Check sheet for the modelled part. Datum: model origin and axes. Units: mm. A direction names the side the tool comes from. Give positions to 0.01 mm unless a question says otherwise; leave off trailing zeros. Order: outer loops, then holes, each group sorted by start corner. A loop starts at its lowest first (then second) coordinate and runs counter-clockwise, first axis right, second up. Notation, with made-up numbers: (30.5, 88) -> (78.5, 88) arc R33 cw to (78.5, 118) -> close; hole circle Ø5 at (47, -36). An arc over 180 degrees is marked (long way). Write each question's results on one line, items separated by ' | '.
Autodesk Inventor part; units mm, degrees
ref_plane "YZ Plane" through (0, 0, 0) normal (1, 0, 0) x (0, 1, 0)
ref_plane "XZ Plane" through (0, 0, 0) normal (0, 1, 0) x (-1, 0, 0)
ref_plane "XY Plane" through (0, 0, 0) normal (0, 0, 1) x (1, 0, 0)
sketch "Boceto1" plane through (0, 0, 0) normal (0, 1, 0) x (-1, 0, 0)
  line L0 (17.5, 45) -> (-17.5, 45)
  line L1 (-22.5, 40) -> (-22.5, -40)
  line L2 (-17.5, -45) -> (17.5, -45)
  line L3 (22.5, -40) -> (22.5, 40)
  line L4 (22.5, 45) -> (-22.5, -45) construction
  line L5 (-22.5, 45) -> (22.5, -45) construction
  arc A0 (22.5, 40) -> (17.5, 45) centre (17.5, 40) ccw
  arc A1 (-17.5, 45) -> (-22.5, 40) centre (-17.5, 40) ccw
  arc A2 (-22.5, -40) -> (-17.5, -45) centre (-17.5, -40) ccw
  arc A3 (17.5, -45) -> (22.5, -40) centre (17.5, -40) ccw
  point P0 (0, 0)
  dimension "d0" = 45
  dimension "d1" = 90
  dimension "d2" = 5
extrude "Extrusión1" add sketch "Boceto1" along normal blind 10
sketch "Boceto2" plane through (0, 10, 0) normal (0, 1, 0) x (1, 0, 0)
  arc A0 (17.5, -45) -> (22.5, -40) centre (17.5, -40) ccw
  line L0 (22.5, -40) -> (22.5, 40)
  arc A1 (22.5, 40) -> (17.5, 45) centre (17.5, 40) ccw
  line L1 (17.5, 45) -> (-17.5, 45)
  arc A2 (-17.5, 45) -> (-22.5, 40) centre (-17.5, 40) ccw
  line L2 (-22.5, 40) -> (-22.5, -40)
  arc A3 (-22.5, -40) -> (-17.5, -45) centre (-17.5, -40) ccw
  line L3 (-17.5, -45) -> (17.5, -45)
  arc A4 (-21.5, -40) -> (-17.5, -44) centre (-17.5, -40) ccw
  line L4 (-21.5, -40) -> (-21.5, 40)
  arc A5 (-17.5, 44) -> (-21.5, 40) centre (-17.5, 40) ccw
  line L5 (-17.5, 44) -> (17.5, 44)
  arc A6 (21.5, 40) -> (17.5, 44) centre (17.5, 40) ccw
  line L6 (21.5, 40) -> (21.5, -40)
  arc A7 (17.5, -44) -> (21.5, -40) centre (17.5, -40) ccw
  line L7 (17.5, -44) -> (-17.5, -44)
  line L8 (-20.5, 40) -> (-20.5, -40)
  arc A8 (-20.5, -40) -> (-17.5, -43) centre (-17.5, -40) ccw
  line L9 (-17.5, -43) -> (17.5, -43)
  arc A9 (17.5, -43) -> (20.5, -40) centre (17.5, -40) ccw
  line L10 (20.5, -40) -> (20.5, 40)
  arc A10 (20.5, 40) -> (17.5, 43) centre (17.5, 40) ccw
  line L11 (17.5, 43) -> (-17.5, 43)
  arc A11 (-17.5, 43) -> (-20.5, 40) centre (-17.5, 40) ccw
  point P0 (0, 0)
  dimension "d5" = 1
  dimension "d6" = 1
extrude "Extrusión2" cut sketch "Boceto2" against normal blind 2 contours L4 A5 L5 A6 L6 A7 L7 A4
sketch "Boceto3" plane through (0, 10, 0) normal (0, 1, 0) x (1, 0, 0)
  line L0 (17.5, 43) -> (-17.5, 43)
  arc A0 (-17.5, 43) -> (-20.5, 40) centre (-17.5, 40) ccw
  line L1 (-20.5, 40) -> (-20.5, -40)
  arc A1 (-20.5, -40) -> (-17.5, -43) centre (-17.5, -40) ccw
  line L2 (-17.5, -43) -> (17.5, -43)
  arc A2 (17.5, -43) -> (20.5, -40) centre (17.5, -40) ccw
  line L3 (20.5, -40) -> (20.5, 40)
  arc A3 (20.5, 40) -> (17.5, 43) centre (17.5, 40) ccw
  point P0 (0, 0)
extrude "Extrusión3" cut sketch "Boceto3" against normal blind 7
sketch "Boceto4" plane through (0, 3, 0) normal (0, 1, 0) x (1, 0, 0)
  circle A0 centre (0, 0) radius 2
  circle A1 centre (0, 0) radius 1.1
  dimension "d11" = 4
  dimension "d12" = 2.2
extrude "Extrusión4" add sketch "Boceto4" along normal blind 5.4
fillet "Empalme1" radius 2 1 edges at (-2, 3, 0)
sketch "Boceto5" plane through (0, 3, 0) normal (0, 1, 0) x (1, 0, 0)
  line L0 (17.5, -43) -> (-17.5, -43) construction
  line L1 (0, -43) -> (0, -37.1) construction
  line L2 (-17.5, 43) -> (17.5, 43) construction
  line L3 (0, 43) -> (0, 37.1) construction
  circle A0 centre (0, -37.1) radius 2
  circle A1 centre (0, -37.1) radius 1.1
  circle A2 centre (0, 37.1) radius 2
  circle A3 centre (0, 37.1) radius 1.1
  point P0 (0, 0)
  dimension "d16" = 5.9
  dimension "d17" = 5.9
  dimension "d18" = 4
  dimension "d19" = 2.2
  dimension "d20" = 4
  dimension "d21" = 2.2
extrude "Extrusión5" add sketch "Boceto5" along normal blind 5.4
fillet "Empalme2" radius 2 2 edges at (-2, 3, 37.1) (-2, 3, -37.1)
sketch "Sketch10" plane through (17.5, 0, -45) normal (0, 0, -1) x (-1, 0, 0)
  line L0 (-3.0024, 10) -> (14.9976, 10)
  line L1 (14.9976, 10) -> (14.9976, 7)
  line L2 (14.9976, 7) -> (-3.0024, 7)
  line L3 (-3.0024, 7) -> (-3.0024, 10)
  point P0 (17.5, 0)
  dimension "d37" = 18
  dimension "d38" = 3
extrude "Extrusion10" cut sketch "Sketch10" against normal blind 5
properties part number "Pieza_baja"
1. Material ranges on probe 1 along X at (y, z) = (5, 0); probe 2 along Z at (x, y) = (10, 3.75); probe 3 along X at (y, z) = (9.5, -0.5), recorded low to high. Write a range as from..to.
Verdict:
probe 1: x = -22.5..-20.5, -2..-1.1, 1.1..2, 20.5..22.5 | probe 2: z = -45..-43, 43..45 | probe 3: x = -22.5..-21.5, 21.5..22.5
2. Gauge pin test, flat ends, axial feed: pin 1 Ø2.5 at (x, z) = (0, -37.5) entering from +Y; pin 2 Ø20.5 at (x, z) = (-9.5, -18) entering from +Y; pin 3 Ø2.5 at (x, z) = (16, -42.5) entering from +Y. Record the tip position at first contact, or that the pin passes through.
Verdict:
pin 1: stops at y = 8.4 | pin 2: stops at y = 3 | pin 3: stops at y = 7
3. Mould release check, pull along X, two halves, no side actions. Record for faces 4 (the flat face through (-22.5, 5, -1)), 5 (the flat face through (22.5, 5, 1)), 6 (the cylindrical face through (0.923, 6.676, 35.326)): +X half, -X half, draft (parallel to the pull), parting line (faces both ways), or undercut.
Verdict:
face 4: -X half | face 5: +X half | face 6: undercut
4. Section check A-A on y = 6. Record the cut outline in (x, z).
Verdict:
outline: (-22.5, -40) arc R5 ccw to (-17.5, -45) -> (17.5, -45) arc R5 ccw to (22.5, -40) -> (22.5, 40) arc R5 ccw to (17.5, 45) -> (-17.5, 45) arc R5 ccw to (-22.5, 40) -> close; circle Ø4 at (0, -37.1); circle Ø4 at (0, 0); circle Ø4 at (0, 37.1); hole (-20.5, -40) arc R3 ccw to (-17.5, -43) -> (17.5, -43) arc R3 ccw to (20.5, -40) -> (20.5, 40) arc R3 ccw to (17.5, 43) -> (-17.5, 43) arc R3 ccw to (-20.5, 40) -> close; hole circle Ø2.2 at (0, -37.1); hole circle Ø2.2 at (0, 0); hole circle Ø2.2 at (0, 37.1)
5. Section check C-C on x = -15.5. Record the cut outline in (y, z).
Verdict:
outline: (0, -45) -> (10, -45) -> (10, -44) -> (8, -44) -> (8, -43) -> (3, -43) -> (3, 43) -> (8, 43) -> (8, 44) -> (10, 44) -> (10, 45) -> (0, 45) -> close
6. Section check D-D on z = 25. Record the cut outline in (x, y).
Verdict:
outline: (-22.5, 0) -> (22.5, 0) -> (22.5, 10) -> (21.5, 10) -> (21.5, 8) -> (20.5, 8) -> (20.5, 3) -> (-20.5, 3) -> (-20.5, 8) -> (-21.5, 8) -> (-21.5, 10) -> (-22.5, 10) -> close
7. Section check B-B on z = -37.1. Record the cut outline in (x, y).
Verdict:
outline: (-22.5, 0) -> (22.5, 0) -> (22.5, 10) -> (21.5, 10) -> (21.5, 8) -> (20.5, 8) -> (20.5, 3) -> (4, 3) arc R2 cw to (2, 5) -> (2, 8.4) -> (1.1, 8.4) -> (1.1, 3) -> (-1.1, 3) -> (-1.1, 8.4) -> (-2, 8.4) -> (-2, 5) arc R2 cw to (-4, 3) -> (-20.5, 3) -> (-20.5, 8) -> (-21.5, 8) -> (-21.5, 10) -> (-22.5, 10) -> close
8. Access from +Z, -Z, +X, -X, +Y, -Y to the whole of each face (thin tool, end or side, straight path). Record for faces 1 (the cylindrical face through (21.07, 4.93, 43.5)), 2 (the flat face through (0, 3, -37)), 3 (the flat face through (2.502, 8.2, -44.2)).
Verdict:
face 1: +Z, +X, +Y, -Y | face 2: +Y | face 3: -Z, +Y
